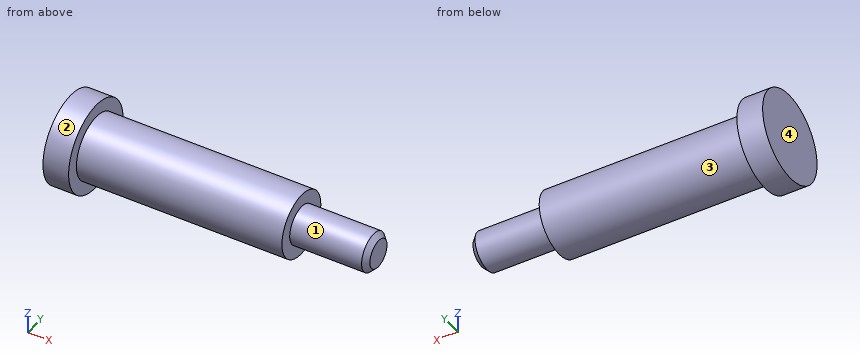
Autodesk Inventor part; units mm, degrees
ref_plane "Начальная плоскость" through (0, 0, 0) normal (1, 0, 0) x (0, 1, 0)
ref_plane "XZ Plane" through (0, 0, 0) normal (0, 1, 0) x (-1, 0, 0)
ref_plane "XY Plane" through (0, 0, 0) normal (0, 0, 1) x (1, 0, 0)
sketch "Основной эскиз" plane through (0, 0, 0) normal (0, 0, 1) x (1, 0, 0)
  line L0 (0, 0) -> (120, 0)
  line L1 (0, 0) -> (0, 17.5)
  line L2 (10, 17.5) -> (10, 12.5)
  line L3 (0, 17.5) -> (10, 17.5)
  line L4 (90, 12.5) -> (90, 7.5)
  line L5 (10, 12.5) -> (90, 12.5)
  line L6 (120, 7.5) -> (120, 0)
  line L7 (90, 7.5) -> (120, 7.5)
  dimension "d3" = 35
  dimension "d4" = 25
  dimension "d5" = 15
revolve "Вращение1" add sketch "Основной эскиз" angle 360 about axis through (0, 0, 0) along (1, 0, 0)
chamfer "Фаска1" distance 2 angle 45 1 edges at (120, -7.5, 0) measured on face at (100, 7.4757, -0.6035)
properties part number "Вал" material "Steel"
Model file for the job. Use its own axes, mm. Face numbers are marked on the shaded views. A direction names the side the tool comes from. Coordinates: 2 decimals unless noted, no trailing zeros. Write each loop counter-clockwise with the first axis right and the second up, starting at its lowest first coordinate (ties: lowest second). Pieces come first, ordered by that corner, then holes. Notation, with made-up numbers: (35.25, 85.25) -> (59.25, 85.25) arc R24 cw to (59.25, 95.25) -> close; hole circle Ø8 at (74, -6). An arc over 180 degrees is marked (long way). One line per item, written item: value. Start each with the question number.
1) Slice it at A-A on y = 0. Write the cut outline in (x, z).
2) Pull direction X, two halves, no side cores. Call the marked faces 3 and 4: +X half, -X half, draft (parallel to the pull), parting line (faces both ways), or undercut.
3) Which spindle directions (+Z, -Z, +X, -X, +Y, -Y) get a long thin tool onto all of the face, cutting with end or side? Do the marked faces 1 and 2. Say none if no direction does.
4) Flat gauge pins, fed straight in: pin 1 Ø1 at (x, y) = (30, 4.5) entering from +Z; pin 2 Ø12.5 at (y, z) = (-2, -5.5) entering from +X; pin 3 Ø1 at (x, z) = (67, -4.5) entering from -Y; pin 4 Ø1 at (x, y) = (69.5, 0) entering from -Z. Where does each tip first touch, or does it go through?
5) Slice it at C-C on x = 59.5. Write the cut outline in (y, z).
6) Probe probe 1 along X at (y, z) = (-7.5, 9); probe 2 along X at (y, z) = (-10.5, -13); probe 3 along Z at (x, y) = (37, -10.5). List the from-to ranges inside material, lowest first.
7) Slice it at D-D on x = 99. Write the cut outline in (y, z), then the cut area to 3 significant figures.
Answers follow:
1. outline: (0, -17.5) -> (10, -17.5) -> (10, -12.5) -> (90, -12.5) -> (90, -7.5) -> (118, -7.5) -> (120, -5.5) -> (120, 5.5) -> (118, 7.5) -> (90, 7.5) -> (90, 12.5) -> (10, 12.5) -> (10, 17.5) -> (0, 17.5) -> close
2. face 3: draft
2. face 4: -X half
3. face 1: +X
3. face 2: +X, -X
4. pin 1: z = 11.84
4. pin 2: x = 120
4. pin 3: y = -11.84
4. pin 4: z = -12.5
5. outline: circle Ø25 at (0, 0)
6. probe 1: 0 to 90
6. probe 2: 0 to 10
6. probe 3: -6.78 to 6.78
7. outline: circle Ø15 at (0, 0)
7. area: 177 mm2
